The model under review builds one solid part; all positions refer to its coordinate system, in mm. Round coordinates to 2 decimals unless told otherwise and drop trailing zeros. Write each loop counter-clockwise with the first axis right and the second up, starting at its lowest first coordinate (ties: lowest second). Pieces come first, ordered by that corner, then holes. Notation, with made-up numbers: (51.5, 45) -> (89.5, 45) arc R6 ccw to (89.5, 56) -> close; hole circle Ø2 at (68.5, 33). An arc over 180 degrees is marked (long way). Answer as a JSON object with one key per item and string values. Group by question number.
1) We need section C-C, the plane y = 190. Write out the cut boundary in (x, z).
2) We need section A-A, the plane z = 175. Write out the cut boundary in (x, y).
3) To check wall thickness, follow probe 1 along Y at (x, z) = (2.5, 136); probe 2 along Z at (x, y) = (0.75, 223.6); probe 3 along Z at (x, y) = (2.25, 165.5). State the ranges of each line that lie inside material, in increasing order. Write a range as [from, to].
4) We need section B-B, the plane x = 2. Write out the cut boundary in (y, z).
5) Insertion check: pin 1 Ø1 at (x, z) = (2, 153) entering from +Y; pin 2 Ø1.5 at (x, z) = (1, 161.5) entering from +Y; pin 3 Ø1 at (x, z) = (1.5, 218) entering from +Y. Each pin has a flat end and moves straight along its axis. Give the tip position at first contact, or say it passes through.
Autodesk Inventor part; units mm, degrees
ref_plane "YZ Plane" through (0, 0, 0) normal (1, 0, 0) x (0, 1, 0)
ref_plane "XZ Plane" through (0, 0, 0) normal (0, 1, 0) x (-1, 0, 0)
ref_plane "XY Plane" through (0, 0, 0) normal (0, 0, 1) x (1, 0, 0)
sketch "Sketch1" plane through (0, 0, 0) normal (1, 0, 0) x (0, 1, 0)
  line L0 (11.6, 259.0874) -> (11.6, 234.0874)
  line L1 (11.6, 234.0874) -> (6, 234.0874)
  line L2 (6, 234.0874) -> (6, 34.0874)
  line L3 (6, 34.0874) -> (11.6, 34.0874)
  line L4 (11.6, 34.0874) -> (11.6, 9.0874)
  line L5 (11.6, 9.0874) -> (253.6, 134.0874)
  line L6 (253.6, 134.0874) -> (11.6, 259.0874)
  circle A0 centre (223.6, 134.0874) radius 2.4
  line L7 (253.6, 134.0874) -> (6, 134.0874) construction
  point P0 (0, 0)
  dimension "d0" = 4.8
  dimension "d1" = 5.6
  dimension "d2" = 200
  dimension "d4" = 30
  dimension "d5" = 250
  dimension "d8" = 242
  dimension "d9" = 212
extrude "Extrusion1" add sketch "Sketch1" along normal blind 3
fillet "Fillet1" radius 10 1 edges at (1.5, 253.6, 134.0874)
sketch "Sketch2" plane through (0, 0, 0) normal (-1, 0, 0) x (0, 0, 1)
  line L0 (46.5951, 27.2148) -> (221.5798, 27.2148)
  line L1 (221.5798, 27.2148) -> (134.0874, 196.6)
  line L2 (134.0874, 196.6) -> (46.5951, 27.2148)
  line L3 (234.0874, 6) -> (34.0874, 6)
  circle A0 centre (134.0874, 223.6) radius 2.4
  line L4 (134.0874, 223.6) -> (134.0874, 6) construction
  line L5 (234.0874, 6) -> (34.0874, 6)
  line L6 (9.0874, 11.6) -> (125.2027, 236.3991)
  point P0 (0, 0)
extrude "Extrusion2" cut sketch "Sketch2" against normal blind 10 contours L2 L1 L0
equation "\"d2\" = SlotLength"
equation "\"d4\" = HingeDistance"
equation "\"d5\" = StandWidth"
equation "\"d13\" = Width"
equation "\"ScrewDiameter\" = 3"
equation "\"Width\" = 10"
equation "\"SlotLength\" = 200"
equation "\"HingeDistance\" = 30"
equation "\"StandWidth\" = 250"
properties part number "Stand" material "ABS Plastic"
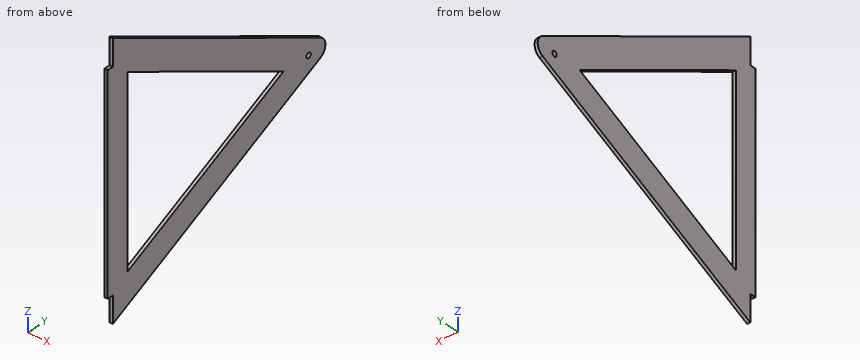
Here are the results:
{
 "1": {"outline": "(0, 101.24) -> (3, 101.24) -> (3, 130.68) -> (0, 130.68) -> close; (0, 137.5) -> (3, 137.5) -> (3, 166.94) -> (0, 166.94) -> close"},
 "2": {"outline": "(0, 6) -> (3, 6) -> (3, 27.21) -> (0, 27.21) -> close; (0, 117.39) -> (3, 117.39) -> (3, 174.39) -> (0, 174.39) -> close"},
 "3": {"probe 1": "y = [6, 27.21], [192.9, 222.15], [225.05, 241.63]", "probe 2": "z = [118.59, 131.69], [136.49, 149.58]", "probe 3": "z = [88.58, 118.02], [150.15, 179.59]"},
 "4": {"outline": "(6, 34.09) -> (11.6, 34.09) -> (11.6, 9.09) -> (236.4, 125.2) arc R10 ccw to (236.4, 142.97) -> (11.6, 259.09) -> (11.6, 234.09) -> (6, 234.09) -> close; hole (27.21, 46.6) -> (196.6, 134.09) -> (27.21, 221.58) -> close; hole circle Ø4.8 at (223.6, 134.09)"},
 "5": {"pin 1": "stops at y = 217.95", "pin 2": "stops at y = 201.98", "pin 3": "stops at y = 92.11"}
}
